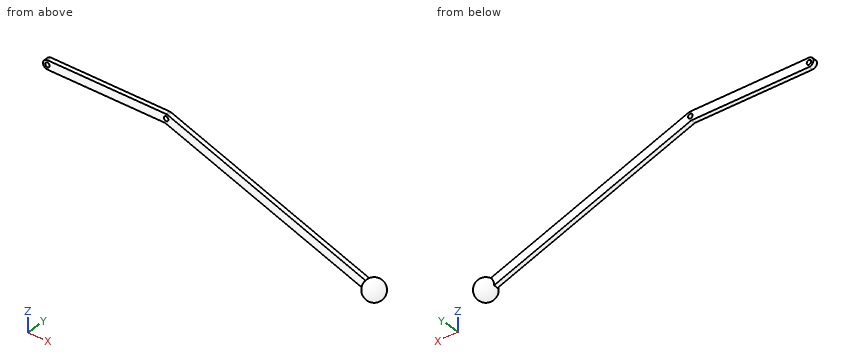
from build123d import *

# Parameters (mm, degrees)
SKETCH1_R           = 5
BOSS_EXTRUDE1_DEPTH = 5
SKETCH2_R           = 5
BOSS_EXTRUDE2_DEPTH = 5


with BuildPart() as part:
    # Sketch1 → Boss-Extrude1 (new, symmetric)
    with BuildSketch(Plane(origin=(0, 0, 0), x_dir=(1, 0, 0), z_dir=(0, 1, 0))):
        with BuildLine():
            ThreePointArc((3.420201433, -9.396926208), (1.736481777, -9.84807753), (0, -10))
            Line((0, -10), (-265, -10))
            ThreePointArc((-265, -10), (-275, 0), (-265, 10))
            Line((-265, 10), (-2.224544129, 9.832109877))
            Line((-2.224544129, 9.832109877), (457.029182752, 176.986796437))
            ThreePointArc((457.029182752, 176.986796437), (469.846310393, 171.010071663), (463.869585618, 158.192944022))
            Line((463.869585618, 158.192944022), (3.420201433, -9.396926208))
        make_face()
        with Locations(Location((460.449384185, 167.58987023, 0), (0, 0, 270))):
            Circle(SKETCH1_R, mode=Mode.SUBTRACT)
        with Locations(Location((0, 0, 0), (0, 0, 270))):
            Circle(SKETCH1_R, mode=Mode.SUBTRACT)
        with Locations(Location((-265, 0, 0), (0, 0, 270))):
            Circle(SKETCH1_R, mode=Mode.SUBTRACT)
    extrude(amount=BOSS_EXTRUDE1_DEPTH, both=True)

    # Sketch2 → Boss-Extrude2 (add, symmetric)
    with BuildSketch(Plane(origin=(0, 0, 0), x_dir=(1, 0, 0), z_dir=(0, 1, 0))):
        with Locations((460.449384185, 167.58987023)):
            Circle(SKETCH2_R)
    extrude(amount=BOSS_EXTRUDE2_DEPTH, both=True)

    # Sketch3 → Revolve1 (revolve)
    with BuildSketch(Plane(origin=(0, 0, 0), x_dir=(1, 0, 0), z_dir=(0, 1, 0))):
        with BuildLine():
            Line((453.692605533, 189.051369298), (467.206162837, 146.128371161))
            ThreePointArc((467.206162837, 146.128371161), (481.910883253, 174.346648881), (453.692605533, 189.051369298))
        make_face()
    revolve(axis=Axis((453.692605533, 0, -189.051369298), (0.30030127341076346, 0, 0.9538444030280169)))


solid = part.part
Can you work these out from the model? Positions are in its coordinate system, mm. Coordinates: 2 decimals unless noted, no trailing zeros. Write each loop counter-clockwise with the first axis right and the second up, starting at its lowest first coordinate (ties: lowest second). Pieces come first, ordered by that corner, then holes. Notation, with made-up numbers: (9.5, 31) - (52.5, 31) arc R18 cw to (52.5, 62) - close; hole circle Ø4 at (-19.5, -36.75). An arc over 180 degrees is marked (long way). Return JSON: item names as keys, results as strings. Group by question number.
Item 1: Please list where these lines run through material, in increasing order: probe 1 along Z at (x, y) = (-265, 0); probe 2 along Z at (x, y) = (-9.5, -2); probe 3 along Z at (x, y) = (209, -1.5).
Item 2: If we section it at A-A (x = -84): Write out the boundary of the cut face in (y, z).
Item 3: I'm going to push flat-ended pins straight in: pin 1 Ø11.5 at (x, z) = (0, 0) entering from -Y; pin 2 Ø3 at (x, y) = (105.5, -1) entering from +Z. Where does each tip first touch, or does it pass through?
Item 4: If we section it at B-B (z = -49.5): Write out the boundary of the cut face in (x, y), then the cut area to 3 significant figures.
Return value:
{
 "1": {"probe 1": "z = -10 to -5, 5 to 10", "probe 2": "z = -9.84 to 10", "probe 3": "z = -86.71 to -65.43"},
 "2": {"outline": "(-5, -9.88) - (5, -9.88) - (5, 10) - (-5, 10) - close"},
 "3": {"pin 1": "stops at y = -5", "pin 2": "stops at z = -27.21"},
 "4": {"outline": "(106.76, -5) - (165.24, -5) - (165.24, 5) - (106.76, 5) - close", "area": "585 mm^2"}
}
